```python
from build123d import *

# Parameters (mm, degrees)
SKETCH1_W           = 42.5
SKETCH1_H           = 42.5
BOSS_EXTRUDE1_DEPTH = 47
SKETCH2_R           = 1
CUT_EXTRUDE1_DEPTH  = 2
SKETCH3_R           = 2.5
BOSS_EXTRUDE2_DEPTH = 22
SKETCH4_R           = 11
BOSS_EXTRUDE3_DEPTH = 2.35


with BuildPart() as part:
    # Sketch1 → Boss-Extrude1 (new body)
    with BuildSketch(Plane.XY):
        Rectangle(SKETCH1_W, SKETCH1_H)
    extrude(amount=BOSS_EXTRUDE1_DEPTH)

    # Sketch2 → Cut-Extrude1 (cut)
    with BuildSketch(Plane.XY.offset(47)):
        with Locations((-15.375, 15.375)):
            Circle(SKETCH2_R)
        with Locations((15.375, 15.375)):
            Circle(SKETCH2_R)
        with Locations((15.375, -15.375)):
            Circle(SKETCH2_R)
        with Locations((-15.375, -15.375)):
            Circle(SKETCH2_R)
    extrude(amount=-CUT_EXTRUDE1_DEPTH, mode=Mode.SUBTRACT)

    # Sketch3 → Boss-Extrude2 (add)
    with BuildSketch(Plane.XY.offset(47)):
        Circle(SKETCH3_R)
    extrude(amount=BOSS_EXTRUDE2_DEPTH)

    # Sketch4 → Boss-Extrude3 (add)
    with BuildSketch(Plane.XY.offset(47)):
        Circle(SKETCH4_R)
    extrude(amount=BOSS_EXTRUDE3_DEPTH)


solid = part.part
```
Input: part model. Units: mm. Frame: model coordinates. A direction names the side the tool comes from. Round coordinates to 2 decimals unless told otherwise and drop trailing zeros. Loops run counter-clockwise (first coordinate to the right, second up) from the corner with the lowest first, then second, coordinate; pieces in that order, holes last.
1) Section query D-D on x = -5. Return the cut outline in (y, z), plus the area to 3 significant figures.
Ans:
outline: (-21.25, 0) - (21.25, 0) - (21.25, 47) - (9.8, 47) - (9.8, 49.35) - (-9.8, 49.35) - (-9.8, 47) - (-21.25, 47) - close
area: 2,040 mm2
2) Material intervals for line 1 (Z direction, x = 19, y = -14.5); line 2 (Z direction, x = 10, y = -1); line 3 (Y direction, x = 2, z = 48.5), sorted ascending.
Ans:
line 1: z = 0 to 47
line 2: z = 0 to 49.35
line 3: y = -10.82 to 10.82
3) Pin query (flat end, axial travel): pin 1 (1 mm diameter, centred on x = 15.5, y = -15, fed in from +Z); pin 2 (2 mm diameter, centred on x = 0, y = -10, fed in from +Z); pin 3 (2 mm diameter, centred on x = -15.5, y = -15, fed in from +Z). Return the tip coordinate at first contact, or that it passes through.
Ans:
pin 1: stops at z = 45
pin 2: stops at z = 49.35
pin 3: stops at z = 47
4) Section query A-A on y = 0. Return the cut outline in (x, z).
Ans:
outline: (-21.25, 0) - (21.25, 0) - (21.25, 47) - (11, 47) - (11, 49.35) - (2.5, 49.35) - (2.5, 69) - (-2.5, 69) - (-2.5, 49.35) - (-11, 49.35) - (-11, 47) - (-21.25, 47) - close
5) Set-up query: faces 1 (the flat face through (0, -21.25, 23)), 2 (the flat face through (-10, -9, 47)). Return all of +Z, -Z, +X, -X, +Y, -Y with unobstructed straight access to the full face (end or side cutting, diameter ignored); none if empty.
Ans:
face 1: +Z, -Z, +X, -X, -Y
face 2: +Z
6) Section query C-C on z = 64. Return the cut outline in (x, y), plus the area to 3 significant figures.
Ans:
outline: circle Ø5 at (0, 0)
area: 19.6 mm2
